```python
from build123d import *

# Parameters (mm, degrees)
BOSS_EXTRU_1_DEPTH = 15
ESQUISSE2_R        = 5
BOSS_EXTRU_2_DEPTH = 75
ESQUISSE3_R        = 7.5
BOSS_EXTRU_3_DEPTH = 5


with BuildPart() as part:
    # Esquisse1 → Boss.-Extru.1 (new body)
    with BuildSketch(Plane.XY):
        Polygon((-0.686649648, 3.395366293), (-3.283798289, 1.103027108), (-2.597148641, -2.292339185), (0.686649648, -3.395366293), (3.283798289, -1.103027108), (2.597148641, 2.292339185), align=None)
    extrude(amount=BOSS_EXTRU_1_DEPTH)

    # Esquisse2 → Boss.-Extru.2 (add)
    with BuildSketch(Plane.XY.offset(15)):
        Circle(ESQUISSE2_R)
    extrude(amount=BOSS_EXTRU_2_DEPTH)

    # Esquisse3 → Boss.-Extru.3 (add)
    with BuildSketch(Plane.XY.offset(90)):
        Circle(ESQUISSE3_R)
    extrude(amount=BOSS_EXTRU_3_DEPTH)


solid = part.part
```
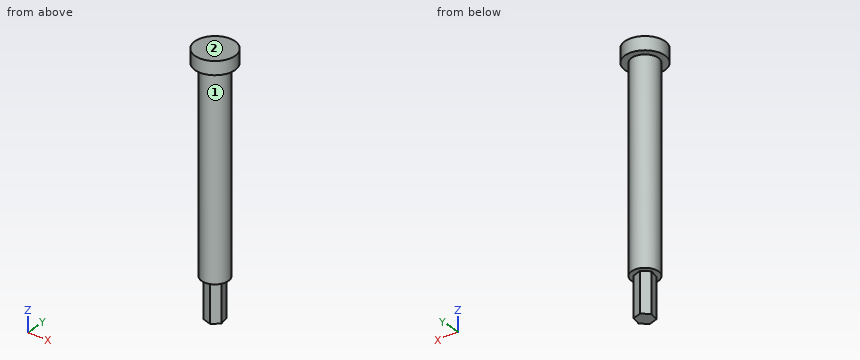
Source: CAD feature listing. Evaluate the final solid. Frame: model axes, mm. Face numbers are marked on the shaded views. A direction names the side the tool comes from. Give positions to 0.01 mm unless a question says otherwise; leave off trailing zeros. Order: outer loops, then holes, each group sorted by start corner. A loop starts at its lowest first (then second) coordinate and runs counter-clockwise, first axis right, second up.
(1) Material intervals for line 1 along Z through (x, y) = (-3, 2.5); line 2 along Z through (x, y) = (2, -6); line 3 along X through (y, z) = (1.25, 36), sorted ascending.
(2) Section query A-A (y = 0). Return the cut outline in (x, z), plus the area to 3 significant figures.
(3) Access query for the marked faces 1 and 2. Directions: +Z, -Z, +X, -X, +Y, -Y. A direction counts if a zero-diameter tool reaches every point of the face in a straight line with its end or side. Return the directions, or none.
(4) Section query D-D (y = 6.5). Return the cut outline in (x, z).
(5) Section query B-B (z = 26). Return the cut outline in (x, y), plus the area to 3 significant figures.
(6) Section query C-C (x = 1.75). Return the cut outline in (y, z), plus the area to 3 significant figures.
(7) Contact query for flat-ended pins moving along their axis: P1, Ø5, axis at x = 5, z = 31.5, coming from the +Y side; P2, Ø8, axis at x = 1, y = 5, coming from the -Z side; P3, Ø5, axis at y = 4, z = 20.5, coming from the -X side; P4, Ø5, axis at y = 0.5, z = 59.5, coming from the +X side. Output: stop coordinate, or through.
Outcome:
1. line 1: z = 15 to 95
1. line 2: z = 90 to 95
1. line 3: x = -4.84 to 4.84
2. outline: (-7.5, 90) - (-5, 90) - (-5, 15) - (-3.06, 15) - (-3.06, 0) - (3.06, 0) - (3.06, 15) - (5, 15) - (5, 90) - (7.5, 90) - (7.5, 95) - (-7.5, 95) - close
2. area: 917 mm2
3. face 1: -Z
3. face 2: +Z, +X, -X, +Y, -Y
4. outline: (-3.74, 90) - (3.74, 90) - (3.74, 95) - (-3.74, 95) - close
5. outline: circle Ø10 at (0, 0)
5. area: 78.5 mm2
6. outline: (-7.29, 90) - (-4.68, 90) - (-4.68, 15) - (-2.46, 15) - (-2.46, 0) - (2.58, 0) - (2.58, 15) - (4.68, 15) - (4.68, 90) - (7.29, 90) - (7.29, 95) - (-7.29, 95) - close
6. area: 851 mm2
7. P1: stops at y = 4.33
7. P2: stops at z = 0
7. P3: stops at x = -4.77
7. P4: stops at x = 5
